Geometry: see drawing. Coordinates: mm, zero at the bounding-box minimum. Give positions to 0.01 mm unless a question says otherwise; leave off trailing zeros. Loops run counter-clockwise (first coordinate to the right, second up) from the corner with the lowest first, then second, coordinate; pieces in that order, holes last. Notation, with made-up numbers: M 71,-21.5 L 80,-21.5 A38 ccw 80,16.5 Z; hole C 3.25,49.25 d4. An arc over 180 degrees is marked long. Return JSON: item names as keys, results as strings. Group by question number.
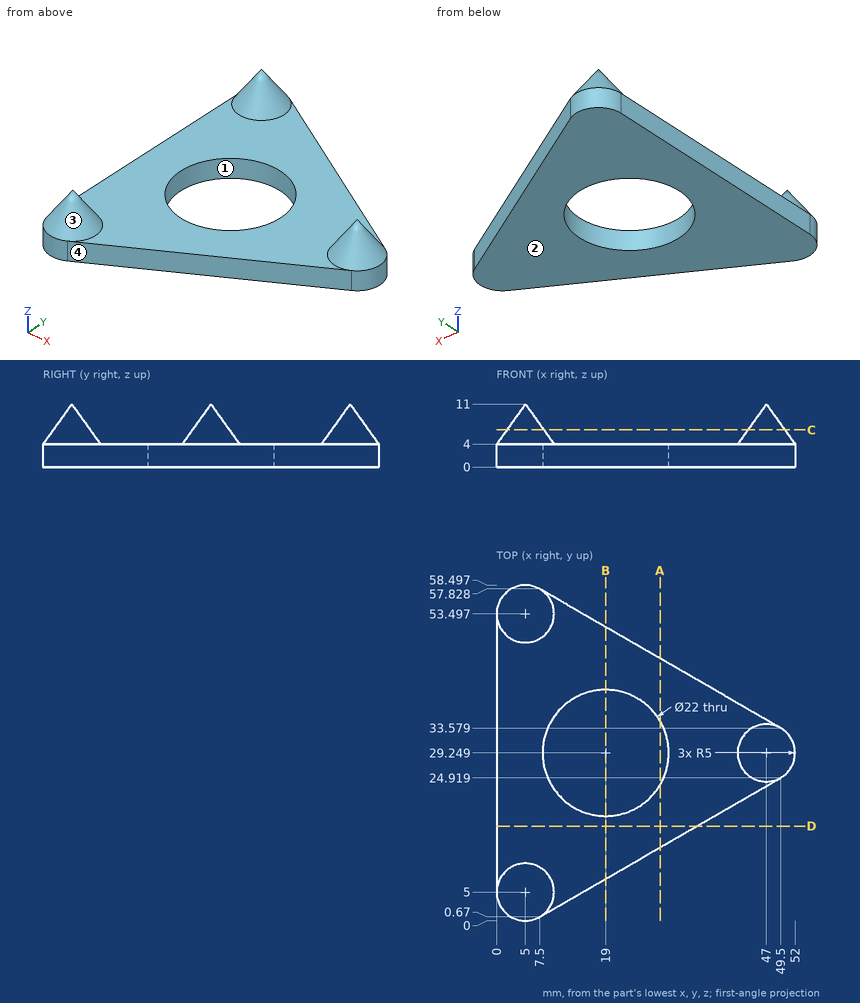
Item 1: Section C-C, the plane z = 6.5. Return loops of the section in (x, y) (1 decimal).
Item 2: Material intervals for line 1 (Z direction, x = 12, y = 4.5); line 2 (Y direction, x = 19, z = 1.7); line 3 (X direction, y = 27.5, z = 2.75) (1 decimal), sorted ascending. Write a range as from..to.
Item 3: Section D-D, the plane y = 16.5. Return loops of the section in (x, z), then the cut area to 3 significant figures.
Item 4: Section B-B, the plane x = 19. Return loops of the section in (y, z).
Item 5: First-contact query: pin 1 Ø1.5 at (x, y) = (45.5, 25) entering from -Z; pin 2 Ø3 at (x, z) = (32.5, 2) entering from -Y; pin 3 Ø25 at (x, y) = (32.5, 38) entering from +Z; pin 4 Ø12 at (x, y) = (40.5, 22.5) entering from +Z. Flat tips, straight axial feed; report the tip coordinate or a pass-through.
Item 6: Section A-A, the plane x = 28.5. Return loops of the section in (y, z) (1 decimal).
Item 7: Pull-direction query (X, two-part tool) for the marked faces 1, 2, 3 and 4; classes: pulls with the +X half, pulls with the -X half, needs draft (parallel to the pull), parting line crosses it, or undercut.
Answer below:
{
 "1": {"outline": "C 5,5 d6.4; C 5,53.5 d6.4; C 47,29.2 d6.4"},
 "2": {"line 1": "0..4", "line 2": "7.31..18.25, 40.25..51.19", "line 3": "0..8.1, 29.9..51.7"},
 "3": {"outline": "M 0,0 L 34.92,0 L 34.92,4 L 0,4 Z", "area": "140 mm^2"},
 "4": {"outline": "M 7.31,0 L 18.25,0 L 18.25,4 L 7.31,4 Z; M 40.25,0 L 51.19,0 L 51.19,4 L 40.25,4 Z"},
 "5": {"pin 1": "z = 0", "pin 2": "y = 14.24", "pin 3": "z = 4.79", "pin 4": "z = 6.28"},
 "6": {"outline": "M 12.8,0 L 23.7,0 L 23.7,4 L 12.8,4 Z; M 34.8,0 L 45.7,0 L 45.7,4 L 34.8,4 Z"},
 "7": {"face 1": "undercut", "face 2": "needs draft", "face 3": "parting line crosses it", "face 4": "pulls with the +X half"}
}
